```python
from build123d import *

# Parameters (mm, degrees)
F0_R     = 38.1
F0_R_2   = 25.4
F1_DEPTH = 105.41
F2_R     = 3.175
F4_SIZE  = 1.6002


with BuildPart() as f1:
    # F0 (on Front) → F1 (new body)
    with BuildSketch(Plane.XZ):
        Circle(F0_R)
        Circle(F0_R_2, mode=Mode.SUBTRACT)
    extrude(amount=F1_DEPTH)

    # F2 (on Top) → F3 (revolve)
    with BuildSketch(Plane.XY):
        with Locations((-27.94, -92.71)):
            Circle(F2_R)
        with Locations((-27.94, -12.7)):
            Circle(F2_R)
    revolve(axis=Axis((0, -105.41, 0), (0, -1, 0)))

    # F4
    f4_edges = [f1.edges().sort_by_distance(p)[0] for p in [
        (-38.1, -105.41, 0),
        (-38.1, 0, 0),
    ]]
    chamfer(f4_edges, length=F4_SIZE)


solid = f1.part
```
Design review of the part built by this model. Coordinates are the model's own, in mm. A direction names the side the tool comes from. Give positions to 0.01 mm unless a question says otherwise; leave off trailing zeros. Order: outer loops, then holes, each group sorted by start corner. A loop starts at its lowest first (then second) coordinate and runs counter-clockwise, first axis right, second up. Notation, with made-up numbers: (14, 64.25) - (50, 64.25) arc R29 cw to (50, 91.25) - close; hole circle Ø9 at (75, 50). An arc over 180 degrees is marked (long way). Use a Markdown table: item, result. Add a question column.
(1) Add section B-B on z = 0. Give the boundary of the cut face in (x, y) (3 decimals).
(2) Machinability: for faces 1 (the face through (-20.157, -52.172, -15.456)), 2 (the face through (-25, 0, -8)), 3 (the face through (-20.157, -99.937, -15.456)), which of the approach directions +Z, -Z, +X, -X, +Y, -Y give a long, thin tool a straight path to every point of the face, cutting with its end or side? Answer none if there is none.
(3) Clearance check with flat-ended pins moving along their axes: P1, Ø8, axis at x = 13, y = -25, coming from the +Z side; P2, Ø1, axis at y = -11, z = 19, coming from the -X side; P3, Ø6, axis at x = -26.5, y = -16.5, coming from the +Z side. State where each tip first meets the part, or that it passes through.
(4) Add section C-C on y = -27. Give the boundary of the cut face in (x, z).
(5) Wall thickness on probe 1 along Z at (x, y) = (0, -3); probe 2 along X at (y, z) = (-94, -8); probe 3 along Z at (x, y) = (21.5, -50): over which ranges is each line inside the solid? List them lowest first. Write a range as [from, to].
(6) Mouldability with a two-part tool opening along X and no side actions: class faces 4 (the face through (-25, -105.41, -8)), 5 (the face through (-30.235, -51.99, -23.183)), 6 (the face through (-20.157, -5.322, -15.456)) as +X half, -X half, draft (parallel to the pull), parting line (faces both ways), or undercut.
(7) Add section A-A on x = 0. Give the boundary of the cut face in (y, z) (3 decimals), then the cut area to 3 significant figures.
Report:
| question | item | result |
|---|---|---|
| 1 | outline | (-38.1, -103.81) - (-36.5, -105.41) - (-25.4, -105.41) - (-25.4, -94.615) arc R3.175 ccw to (-25.4, -90.805) - (-25.4, -14.605) arc R3.175 ccw to (-25.4, -10.795) - (-25.4, 0) - (-36.5, 0) - (-38.1, -1.6) - close; (25.4, -105.41) - (36.5, -105.41) - (38.1, -103.81) - (38.1, -1.6) - (36.5, 0) - (25.4, 0) - (25.4, -10.795) arc R3.175 ccw to (25.4, -14.605) - (25.4, -90.805) arc R3.175 ccw to (25.4, -94.615) - close |
| 2 | face 1 | none |
| 2 | face 2 | +Z, -Z, +X, -X, +Y |
| 2 | face 3 | -Y |
| 3 | P1 | stops at z = 37.02 |
| 3 | P2 | stops at x = -33.31 |
| 3 | P3 | stops at z = 29.99 |
| 4 | outline | circle Ø76.2 at (0, 0); hole circle Ø50.8 at (0, 0) |
| 5 | probe 1 | z = [-38.1, -25.4], [25.4, 38.1] |
| 5 | probe 2 | x = [-37.25, -23.73], [23.73, 37.25] |
| 5 | probe 3 | z = [-31.45, -13.52], [13.52, 31.45] |
| 6 | face 4 | draft |
| 6 | face 5 | parting line |
| 6 | face 6 | undercut |
| 7 | outline | (-105.41, -36.5) - (-103.81, -38.1) - (-1.6, -38.1) - (0, -36.5) - (0, -25.4) - (-10.795, -25.4) arc R3.175 ccw to (-14.605, -25.4) - (-90.805, -25.4) arc R3.175 ccw to (-94.615, -25.4) - (-105.41, -25.4) - close; (-105.41, 25.4) - (-94.615, 25.4) arc R3.175 ccw to (-90.805, 25.4) - (-14.605, 25.4) arc R3.175 ccw to (-10.795, 25.4) - (0, 25.4) - (0, 36.5) - (-1.6, 38.1) - (-103.81, 38.1) - (-105.41, 36.5) - close |
| 7 | area | 2,680 mm² |
